For this review, take the finished solid that the model builds, in its own axes (mm). A direction names the side the tool comes from. Round coordinates to 2 decimals unless told otherwise and drop trailing zeros. Loops run counter-clockwise (first coordinate to the right, second up) from the corner with the lowest first, then second, coordinate; pieces in that order, holes last.
1) Tool access review of faces 4 (the flat face through (1.4, 0, 0)), 5 (the flat face through (0, 0, -8)), 6 (the flat face through (0.87, 0.49, 1.8)): name each direction out of +Z, -Z, +X, -X, +Y, -Y from which nothing blocks a thin tool from reaching the whole face with its end or side.
2) Wall thickness on L1, parallel to Z at x = -0.5, y = 2.5; L2, parallel to Z at x = 0.5, y = 0.25 (3 decimals); L3, parallel to Y at x = -0.5, z = 1.5: over which ranges is each line inside the solid? List them lowest first.
3) Insertion check: pin 1 (2 mm diameter, centred on x = -0.5, z = 0.5, fed in from -Y); pin 2 (3 mm diameter, centred on x = 1, z = -2.5, fed in from -Y); pin 3 (2 mm diameter, centred on y = -2.5, z = 1, fed in from -X). Each pin has a flat end and moves straight along its axis. Give the tip position at first contact, or say it passes through.
4) Mouldability with a two-part tool opening along Y and no side actions: class faces 1 (the flat face through (1, -1, 2.5)), 2 (the cylindrical face through (-2.579, -1.978, 0.924)), 3 (the flat face through (0.86, -0.51, 1.8)) as pulls with the +Y half, pulls with the -Y half, needs draft (parallel to the pull), parting line crosses it, or undercut.
5) Take a section at A-A (z = -7). State the section outline as (x, y) points.
```python
from build123d import *

# Parameters (mm, degrees)
F_0000_CYLINDER_SKETCH_R    = 3.25
F_0000_CYLINDER_DEPTH       = 2.5
F_0001_FILLET_R             = 0.625
F_0002_EXTRUDE_DEPTH        = 1.385
F_0002_EXTRUDE_ROTATE_ANGLE = 120
F_0005_CYLINDER_SKETCH_R    = 1.2
F_0005_CYLINDER_DEPTH       = 7.7
F_0006_CONE_ROTATE_ANGLE    = 90


with BuildPart() as part:
    # 0000_cylinder_Sketch → 0000_cylinder (new body)
    with BuildSketch(Plane.XY):
        Circle(F_0000_CYLINDER_SKETCH_R)
    extrude(amount=F_0000_CYLINDER_DEPTH)

    # 0001_fillet
    f_0001_fillet_edges = [part.edges().sort_by_distance(p)[0] for p in [
        (-3.25, 0, 2.5),
    ]]
    fillet(f_0001_fillet_edges, radius=F_0001_FILLET_R)


with BuildPart() as body_2:
    # 0002_extrude_Sketch → 0002_extrude (new body)
    with BuildSketch(Plane.XY):
        Polygon((0, 0), (1.154700538, 0), (1.732050808, 1), (1.154700538, 2), (0, 2), (-0.577350269, 1), align=None)
    extrude(amount=F_0002_EXTRUDE_DEPTH)


with BuildPart() as body_2_1:
    # 0002_extrude_Rotate: read off the stored shape, not the designer's step
    # 0002_extrude_Rotate: moved
    add(body_2.part.rotate(Axis((0, 0, 0), (0, 0, 1)), F_0002_EXTRUDE_ROTATE_ANGLE))


with BuildPart() as body_2_2:
    # 0002_extrude_Translate: moved
    add(body_2_1.part.moved(Location((1.154700538, 0, 1.125))))


with BuildPart() as part_1:
    add(part.part)

    # 0004_sub: cut body 2
    add(body_2_2.part, mode=Mode.SUBTRACT)


with BuildPart() as body_2_2_1:
    # 0005_cylinder_Sketch → 0005_cylinder (new body)
    with BuildSketch(Plane.XY):
        with Locations(Location((0, 0, 0), (0, 0, 180))):
            Circle(F_0005_CYLINDER_SKETCH_R)
    extrude(amount=F_0005_CYLINDER_DEPTH)


with BuildPart() as body_2_2_2:
    # 0005_cylinder_Translate: moved
    add(body_2_2_1.part.moved(Location((0, 0, -7.7))))


with BuildPart() as body_3:
    # 0006_cone_Sketch → 0006_cone (revolve)
    with BuildSketch(Plane.XY, mode=Mode.PRIVATE) as f_0006_cone_sk:
        Polygon((0, 0), (1.2, 0), (0.9, 0.3), (0, 0.3), align=None)
    revolve(f_0006_cone_sk.sketch.rotate(Axis((0, -100, 0), (0, 1, 0)), 90), axis=Axis((0, -100, 0), (0, 1, 0)))


with BuildPart() as body_3_1:
    # 0006_cone_Rotate: moved
    add(body_3.part.rotate(Axis((0, 0, 0), (1, 0, 0)), F_0006_CONE_ROTATE_ANGLE))


with BuildPart() as body_3_2:
    # 0006_cone_Translate: moved
    add(body_3_1.part.moved(Location((0, 0, -8))))


with BuildPart() as body_2_2_3:
    add(body_2_2_2.part)

    # 0008_add: union body 3
    add(body_3_2.part)


with BuildPart() as part_2:
    add(part_1.part)

    # 0009_add: union body 2 2
    add(body_2_2_3.part)


solid = part_2.part
```
Response:
1. face 4: -Z
1. face 5: -Z, +X, -X, +Y, -Y
1. face 6: +Z
2. L1: z = 0 to 2.5
2. L2: z = -8 to 1.125
2. L3: y = -3.21 to -1, 1 to 3.21
3. pin 1: stops at y = -3.25
3. pin 2: stops at y = -1.2
3. pin 3: stops at x = -2.88
4. face 1: needs draft
4. face 2: parting line crosses it
4. face 3: undercut
5. outline: circle Ø2.4 at (0, 0)
